Work out the finished part from the listing and answer in its coordinate system (mm). Face numbers are marked on the shaded views. Coordinates: 2 decimals unless noted, no trailing zeros. Write each loop counter-clockwise with the first axis right and the second up, starting at its lowest first coordinate (ties: lowest second). Pieces come first, ordered by that corner, then holes. Notation, with made-up numbers: (16.5, -5) - (57.5, -5) arc R23 cw to (57.5, 16) - close; hole circle Ø2 at (18.25, -27.5). An arc over 180 degrees is marked (long way). Use one line per item in the form item = value. Start each with the question number.
Item 1: A cutting plane is placed at D-D (z = 76). Write down the section's boundary in (x, y).
Item 2: A cutting plane is placed at C-C (x = -89.5). Write down the section's boundary in (y, z), then the cut area to 3 significant figures.
Item 3: A cutting plane is placed at A-A (z = 101.5). Write down the section's boundary in (x, y).
Item 4: A cutting plane is placed at B-B (y = 38.5). Write down the section's boundary in (x, z).
Item 5: Determine the mould class of the marked faces 1, 2 and 3 for opening direction Z: released by +Z, released by -Z, zero draft, split by the parting line, or undercut.
Item 6: Given pin 1 (2 mm diameter, centred on x = 81, y = 44.5, fed in from +Z); pin 2 (5 mm diameter, centred on x = 127, z = -69.5, fed in from +Y), each flat-ended and moving along its own axis, determine where each tip first touches the part or whether it passes through.
Item 7: Consider probe 1 along Y at (x, z) = (-33, 97); probe 2 along Z at (x, y) = (-69, 30); probe 3 along Y at (x, z) = (31.5, -74.5). Determine where each line is inside the solid, lowest interval first.
from build123d import *

# Parameters (mm, degrees)
SKETCH1_W               = 393.7
SKETCH1_H               = 229.108
BASE_FLANGE1_DEPTH      = 2.54
MITER_START             = -196.85
MITER_FLANGE1_DEPTH     = 393.7
MITER_FLANGE1_2_DEPTH   = 393.7
FILLET1_R               = 2.54
F_1_4_CLEARANCE_HOLE1_D = 6.5278


# Read off the part's stored shape, not the designer's step: Miter Flange1
# Sheet-metal steps are written as plain solids
with BuildPart() as part:
    # Sketch1 → Base-Flange1 (new body)
    with BuildSketch(Plane(origin=(0, 0, 0), x_dir=(1, 0, 0), z_dir=(0, 1, 0))):
        Rectangle(SKETCH1_W, SKETCH1_H)
    extrude(amount=-BASE_FLANGE1_DEPTH)

    # Miter Flange1 outline → Miter Flange1 (cut)
    with BuildSketch(Plane.YZ.offset(MITER_START)):
        with BuildLine():
            Line((-2.54, -114.554), (-2.456130493, -114.554))
            ThreePointArc((-2.456130493, -114.554), (-2.518965104, -114.188079664), (-2.54, -113.8174))
            Line((-2.54, -113.8174), (-2.54, -114.554))
        make_face()
    miter_flange1 = extrude(amount=MITER_FLANGE1_DEPTH, mode=Mode.SUBTRACT)

    # Miter Flange1 2 outline → Miter Flange1 2 (add)
    with BuildSketch(Plane.YZ.offset(MITER_START)):
        with BuildLine():
            Line((45.72, -113.8174), (45.72, -92.329))
            Line((45.72, -92.329), (43.18, -92.329))
            Line((43.18, -92.329), (43.18, -113.8174))
            ThreePointArc((43.18, -113.8174), (42.964254855, -114.338254855), (42.4434, -114.554))
            Line((42.4434, -114.554), (0.7366, -114.554))
            ThreePointArc((0.7366, -114.554), (0.215745145, -114.338254855), (0, -113.8174))
            Line((0, -113.8174), (0, -114.554))
            Line((0, -114.554), (-2.456130493, -114.554))
            ThreePointArc((-2.456130493, -114.554), (-1.303322057, -116.381542266), (0.7366, -117.094))
            Line((0.7366, -117.094), (42.4434, -117.094))
            ThreePointArc((42.4434, -117.094), (44.760306079, -116.134306079), (45.72, -113.8174))
        make_face()
    miter_flange1_2 = extrude(amount=MITER_FLANGE1_2_DEPTH)

    # Mirror1: Miter Flange1, Miter Flange1 2 across plane
    add(miter_flange1.mirror(Plane.XY), mode=Mode.SUBTRACT)
    add(miter_flange1_2.mirror(Plane.XY))

    # Fillet1
    fillet1_edges = [part.edges().sort_by_distance(p)[0] for p in [
        (-196.85, 44.45, -92.329),
        (196.85, 44.45, -92.329),
        (-196.85, 44.45, 92.329),
        (196.85, 44.45, 92.329),
    ]]
    fillet(fillet1_edges, radius=FILLET1_R)

    # 1/4 Clearance Hole1 (through all)
    with Locations(Plane(origin=(0, -2.54, 0), x_dir=(-1, 0, 0), z_dir=(0, -1, 0))):
        with Locations((-47.625, -47.625), (-47.625, 47.625), (47.625, 47.625), (47.625, -47.625)):
            Hole(F_1_4_CLEARANCE_HOLE1_D / 2)


solid = part.part
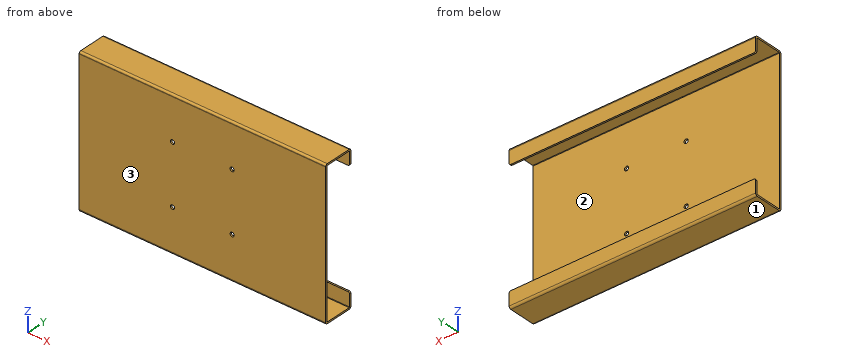
Answer:
q1.outline = (-196.85, -2.54) - (196.85, -2.54) - (196.85, 0) - (-196.85, 0) - close
q2.outline = (-2.54, -113.82) arc R3.28 ccw to (0.74, -117.09) - (42.44, -117.09) arc R3.28 ccw to (45.72, -113.82) - (45.72, -92.33) - (43.18, -92.33) - (43.18, -113.82) arc R0.74 cw to (42.44, -114.55) - (0.74, -114.55) arc R0.74 cw to (0, -113.82) - (0, 113.82) arc R0.74 cw to (0.74, 114.55) - (42.44, 114.55) arc R0.74 cw to (43.18, 113.82) - (43.18, 92.33) - (45.72, 92.33) - (45.72, 113.82) arc R3.28 ccw to (42.44, 117.09) - (0.74, 117.09) arc R3.28 ccw to (-2.54, 113.82) - close
q2.area = 931 mm²
q3.outline = (-196.85, -2.54) - (196.85, -2.54) - (196.85, 0) - (-196.85, 0) - close; (-196.85, 43.18) - (196.85, 43.18) - (196.85, 45.72) - (-196.85, 45.72) - close
q4.outline = (-196.85, -117.09) - (196.85, -117.09) - (196.85, -114.55) - (-196.85, -114.55) - close; (-196.85, 114.55) - (196.85, 114.55) - (196.85, 117.09) - (-196.85, 117.09) - close
q5.face_1 = released by -Z
q5.face_2 = undercut
q5.face_3 = zero draft
q6.pin_1 = 116.92
q6.pin_2 = 0
q7.probe_1 = -2.54 to 0, 43.18 to 45.72
q7.probe_2 = -117.09 to -114.55, 114.55 to 117.09
q7.probe_3 = -2.54 to 0
